```python
from build123d import *
from build123d.topology import SkipClean

# Parameters (mm, degrees)
SKETCH3_R           = 12.5
BOSS_EXTRUDE1_DEPTH = 10
CUT_EXTRUDE3_DEPTH  = 2.5
SKETCH7_R           = 1.500000283
SKETCH7_R_2         = 1.5
CUT_EXTRUDE4_DEPTH  = 20.403607912
SKETCH8_R           = 2.9
CUT_EXTRUDE5_DEPTH  = 4.5


with BuildPart() as part:
    # Sketch3 → Boss-Extrude1 (new body)
    with BuildSketch(Plane(origin=(0, 0, 0), x_dir=(1, 0, 0), z_dir=(0, 1, 0))):
        with Locations(Location((0, 0, 0), (0, 0, 270))):
            Circle(SKETCH3_R)
    extrude(amount=BOSS_EXTRUDE1_DEPTH)

    # Sketch5 → Cut-Extrude3 (cut)
    with BuildSketch(Plane(origin=(0, 2, 0), x_dir=(-1, 0, 0), z_dir=(0, -1, 0))):
        with BuildLine():
            ThreePointArc((7.910254038, -6.299038106), (9.959292144, -5.75), (9.410254038, -3.700961894))
            Line((9.410254038, -3.700961894), (5.080127019, -1.200961894))
            ThreePointArc((5.080127019, -1.200961894), (3.031088913, -1.75), (3.580127019, -3.799038106))
            Line((3.580127019, -3.799038106), (7.910254038, -6.299038106))
        make_face()
        with BuildLine():
            Line((1.5, 0), (1.5, 4.999998598))
            ThreePointArc((1.5, 4.999998598), (0, 6.499998598), (-1.5, 4.999998598))
            Line((-1.5, 4.999998598), (-1.5, 1.154700538))
            ThreePointArc((-1.5, 1.154700538), (-1.566987298, 0.904700538), (-1.75, 0.721687836))
            Line((-1.75, 0.721687836), (-5.080127019, -1.200961894))
            ThreePointArc((-5.080127019, -1.200961894), (-5.629165611, -3.250000029), (-3.580127396, -3.799038324))
            Line((-3.580127396, -3.799038324), (0.75, -1.299038106))
            ThreePointArc((0.75, -1.299038106), (1.299038106, -0.75), (1.5, 0))
        make_face()
    extrude(amount=-CUT_EXTRUDE3_DEPTH, mode=Mode.SUBTRACT)

    # Sketch7 → Cut-Extrude4 (cut, through all)
    with SkipClean():  # the faces are left unmerged after this step: merging them gives an invalid solid
        with BuildSketch(Plane(origin=(0, 2, 0), x_dir=(-1, 0, 0), z_dir=(0, -1, 0))):
            with Locations(Location((0, 4.999998598, 0), (0, 0, 90))):
                Circle(SKETCH7_R)
            with Locations(Location((-4.330127396, -2.500000218, 0), (0, 0, 90))):
                Circle(SKETCH7_R_2)
            with Locations(Location((0, 0, 0), (0, 0, 90))):
                Circle(SKETCH7_R_2)
            with Locations(Location((8.660254038, -5, 0), (0, 0, 90))):
                Circle(SKETCH7_R_2)
            with Locations(Location((4.330127019, -2.5, 0), (0, 0, 90))):
                Circle(SKETCH7_R_2)
        extrude(amount=CUT_EXTRUDE4_DEPTH, mode=Mode.SUBTRACT)

    # Sketch8 → Cut-Extrude5 (cut)
    with SkipClean():  # the faces are left unmerged after this step: merging them gives an invalid solid
        with BuildSketch(Plane(origin=(0, 10, 0), x_dir=(1, 0, 0), z_dir=(0, 1, 0))):
            with Locations(Location((0, 0, 0), (0, 0, 270))):
                Circle(SKETCH8_R)
        extrude(amount=-CUT_EXTRUDE5_DEPTH, mode=Mode.SUBTRACT)

    # Sketch9 → Cut-Revolve1 (revolve, cut)
    with SkipClean():  # the faces are left unmerged after this step: merging them gives an invalid solid
        with BuildSketch(Plane.XY, mode=Mode.PRIVATE) as cut_revolve1_sk:
            with BuildLine():
                Line((21.498533976, 15.074260083), (4.4, 15.074260083))
                Line((4.4, 15.074260083), (4.4, 8))
                ThreePointArc((4.4, 8), (4.985786438, 6.585786438), (6.4, 6))
                Line((6.4, 6), (21.498533976, 6))
                Line((21.498533976, 6), (21.498533976, 15.074260083))
            make_face()
        revolve(cut_revolve1_sk.sketch.rotate(Axis((0, -2.172857957, 0), (0, 1, 0)), 90), axis=Axis((0, -2.172857957, 0), (0, 1, 0)), mode=Mode.SUBTRACT)


solid = part.part
```
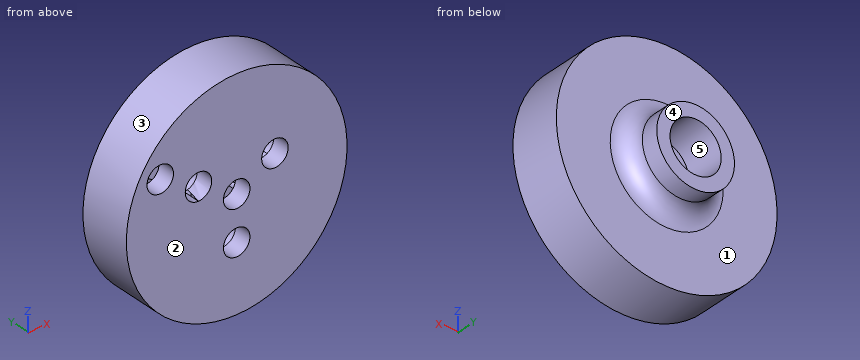
Design review of the part built by this model. Coordinates are the model's own, in mm. Face numbers are marked on the shaded views. A direction names the side the tool comes from. Coordinates: 2 decimals unless noted, no trailing zeros. Order: outer loops, then holes, each group sorted by start corner. A loop starts at its lowest first (then second) coordinate and runs counter-clockwise, first axis right, second up. Notation, with made-up numbers: M 79.5,80 L 112.5,80 A32 ccw 112.5,115 Z; hole C 57,69 d6. An arc over 180 degrees is marked long. Answer as a JSON object with one key per item and string values. Group by question number.
1) Add section C-C, the plane y = 1.25. Write out the cut boundary in (x, z).
2) Add section D-D, the plane z = 7. Write out the cut boundary in (x, y), then the cut area to 3 significant figures.
3) Add section A-A, the plane x = 0. Write out the cut boundary in (y, z).
4) Tool access review of the marked faces 1 and 2: name each direction out of +Z, -Z, +X, -X, +Y, -Y from which nothing blocks a thin tool from reaching the whole face with its end or side.
5) Mouldability with a two-part tool opening along X and no side actions: class the marked faces 3, 4 and 5 as pulls with the +X half, pulls with the -X half, needs draft (parallel to the pull), parting line crosses it, or undercut.
6) For pin 1 (8 mm diameter, centred on x = -9, z = -6, fed in from +Y); pin 2 (5 mm diameter, centred on x = 0, z = 0, fed in from +Y); pin 3 (4 mm diameter, centred on y = 7.5, z = -6, fed in from -X), all flat-tipped, find the tip position at first contact; note any pin that passes through.
7) Wall thickness on L1, parallel to Z at x = 0, y = 0.6; L2, parallel to X at y = 0.5, z = 2.5; L3, parallel to Y at x = -6.5, z = 5: over which ranges is each line inside the solid? List them lowest first.
8) Add section B-B, the plane y = 9.5. Write out the cut boundary in (x, z), then the cut area to 3 significant figures.
Computed values:
{
 "1": {"outline": "C 0,0 d25; hole C -8.66,5 d3; hole C -4.33,2.5 d3; hole C 0,-5 d3; hole C 0,0 d3; hole C 4.33,2.5 d3"},
 "2": {"outline": "M -10.36,0 L 10.36,0 L 10.36,6 L -10.36,6 Z", "area": "124 mm^2"},
 "3": {"outline": "M 0,-12.5 L 6,-12.5 L 6,-6.4 A2 cw 8,-4.4 L 10,-4.4 L 10,-2.9 L 5.5,-2.9 L 5.5,2.9 L 10,2.9 L 10,4.4 L 8,4.4 A2 cw 6,6.4 L 6,12.5 L 0,12.5 L 0,1.5 L 2,1.5 L 2,1.73 L 4.5,1.73 L 4.5,-6.5 L 0,-6.5 Z; M 0,-3.5 L 2,-3.5 L 2,-1.5 L 0,-1.5 Z"},
 "4": {"face 1": "+Y", "face 2": "+Z, -Z, +X, -X, -Y"},
 "5": {"face 3": "parting line crosses it", "face 4": "needs draft", "face 5": "undercut"},
 "6": {"pin 1": "stops at y = 6", "pin 2": "stops at y = 5.5", "pin 3": "stops at x = -11.59"},
 "7": {"L1": "z = -12.5 to -6.5, -3.5 to -1.5, 1.5 to 12.5", "L2": "x = -12.25 to -5.83, -2.83 to 2.83, 5.83 to 12.25", "L3": "y = 0 to 2, 4.5 to 6"},
 "8": {"outline": "C 0,0 d8.8; hole C 0,0 d5.8", "area": "34.4 mm^2"}
}
